Geometry: see drawing. Coordinates: mm, zero at the bounding-box minimum. A direction names the side the tool comes from. Round coordinates to 2 decimals unless told otherwise and drop trailing zeros. Write each loop counter-clockwise with the first axis right and the second up, starting at its lowest first coordinate (ties: lowest second). Pieces come first, ordered by that corner, then holes.
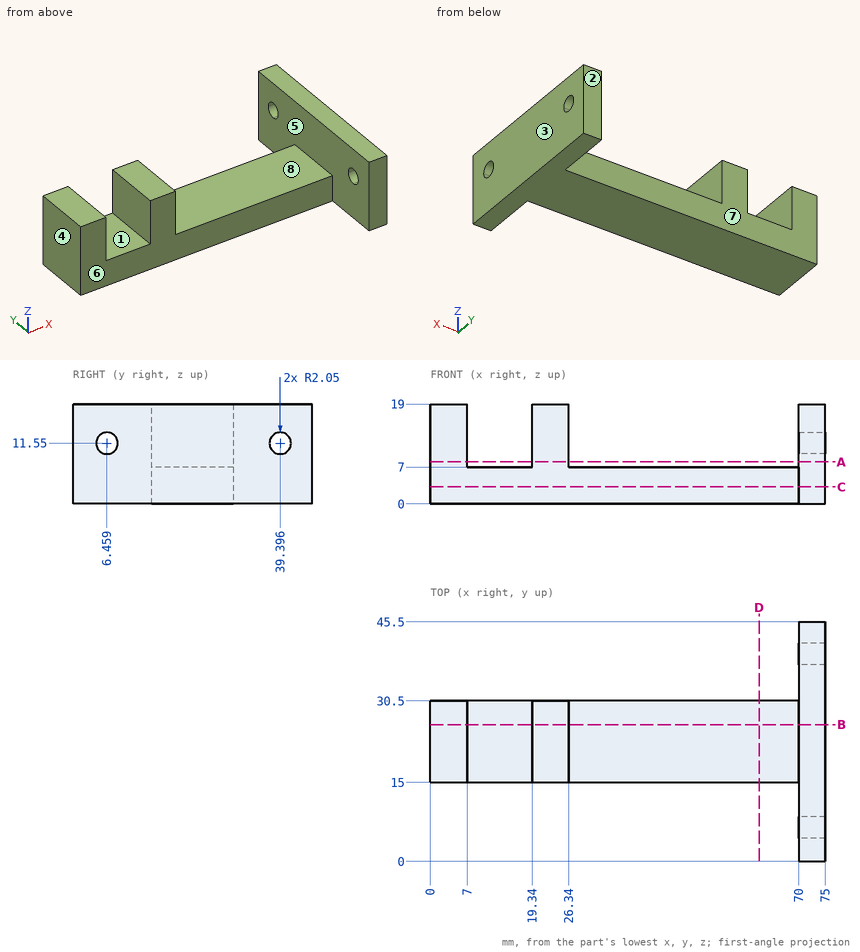
Q1. Section query A-A, the plane z = 8. Output: boundary loops of the cut face in (x, y).
Q2. Line query: line 1 (X direction, y = 30, z = 16); line 2 (X direction, y = 7, z = 6); line 3 (Z direction, x = 39, y = 25). Output: solid intervals per line, ascending.
Q3. Section query D-D, the plane x = 62.5. Output: boundary loops of the cut face in (y, z), and give its area (4 significant figures).
Q4. Section query B-B, the plane y = 26. Output: boundary loops of the cut face in (x, z).
Q5. Pin query (flat end, axial travel): P1, Ø9.5, axis at x = 20, z = 13, coming from the +Y side; P2, Ø12.5, axis at x = 39, y = 21, coming from the +Z side; P3, Ø2, axis at x = 41, z = 7, coming from the -Y side. Return the tip coordinate at first contact, or that it passes through.
Q6. Section query C-C, the plane z = 3.25. Output: boundary loops of the cut face in (x, y), and give its area (3 significant figures).
Q7. Set-up query: the marked faces 5, 6, 7 and 8. Return all of +Z, -Z, +X, -X, +Y, -Y with unobstructed straight access to the full face (end or side cutting, diameter ignored); none if empty.
Q8. Mould query, pull axis X, two halves, no side actions, for the marked faces 1, 2, 3 and 4. Classes: pulls with the +X half, pulls with the -X half, needs draft (parallel to the pull), parting line crosses it, or undercut.
Filled in:
1. outline: (0, 15) - (7, 15) - (7, 30.5) - (0, 30.5) - close; (19.34, 15) - (26.34, 15) - (26.34, 30.5) - (19.34, 30.5) - close; (70, 0) - (75, 0) - (75, 45.5) - (70, 45.5) - close
2. line 1: x = 0 to 7, 19.34 to 26.34, 70 to 75
2. line 2: x = 70 to 75
2. line 3: z = 0 to 7
3. outline: (15, 0) - (30.5, 0) - (30.5, 7) - (15, 7) - close
3. area: 108.5 mm2
4. outline: (0, 0) - (75, 0) - (75, 19) - (70, 19) - (70, 7) - (26.34, 7) - (26.34, 19) - (19.34, 19) - (19.34, 7) - (7, 7) - (7, 19) - (0, 19) - close
5. P1: stops at y = 30.5
5. P2: stops at z = 7
5. P3: stops at y = 15
6. outline: (0, 15) - (70, 15) - (70, 0) - (75, 0) - (75, 45.5) - (70, 45.5) - (70, 30.5) - (0, 30.5) - close
6. area: 1,310 mm2
7. face 5: +Z
7. face 6: +Z, -Z, -X, -Y
7. face 7: +Z, -Z, -X, +Y
7. face 8: +Z, +Y, -Y
8. face 1: undercut
8. face 2: needs draft
8. face 3: pulls with the +X half
8. face 4: pulls with the -X half
